```python
from build123d import *

# Parameters (mm, degrees)
CONG_1_R                     = 1
ENL_V_MAT_EXTRU_1_REACH      = 29.308
R_P_TITION_CIRCULAIRE2_COUNT = 3
R_P_TITION_CIRCULAIRE2_ANGLE = 180
ENL_V_START                  = -3.5
ENL_V_MAT_EXTRU_2_DEPTH      = 3.5
TROU_TARAUD_M3X0_52_D        = 2.5


with BuildPart() as part:
    # Esquisse3 → Révolution1 (revolve)
    with BuildSketch(Plane.XY):
        Polygon((-12.974994046, -8.820980619), (-12.974994046, -3.820980619), (-11.974994046, -3.820980619), (-11.974994046, -5.320980619), (-4.974994046, -5.320980619), (-4.974994046, -3.320980619), (-3.974994046, -3.320980619), (-3.974994046, 9.179019381), (-2.974994046, 9.179019381), (-2.974994046, 5.770549628), (-1.974994046, 5.770549628), (-1.974994046, -4.820980619), (-2.974994046, -4.820980619), (-2.974994046, -8.820980619), align=None)
    revolve(axis=Axis((1.025005954, 13.743921907, 0), (0, -1, 0)))

    # Congé1
    cong_1_edges = [part.edges().sort_by_distance(p)[0] for p in [
        (15.025005954, -8.820980619, 0),
    ]]
    fillet(cong_1_edges, radius=CONG_1_R)

    # Enlèv. mat.-Extru.1: up to this face of the body (flat: up to its plane)
    enl_v_mat_extru_1_end = Plane(part.part.faces().sort_by_distance((13.657310428, -5.320980619, 0))[0])
    # Esquisse5 → Enlèv. mat.-Extru.1 (cut, up to the picked face)
    with BuildSketch(Plane.XZ.offset(8.820980619), mode=Mode.PRIVATE) as enl_v_mat_extru_1_sk1:
        with BuildLine():
            Line((13.674116595, 3), (10.546683691, 3))
            ThreePointArc((10.546683691, 3), (7.546683691, 0), (10.546683691, -3))
            Line((10.546683691, -3), (13.674116595, -3))
            Line((13.674116595, -3), (14.699800285, -3))
            Line((14.699800285, -3), (15.031061769, -3))
            ThreePointArc((15.031061769, -3), (15.351470019, 0), (15.031061769, 3))
            Line((15.031061769, 3), (14.699800285, 3))
            Line((14.699800285, 3), (13.674116595, 3))
        make_face()
    enl_v_mat_extru_1_tool1 = split(extrude(enl_v_mat_extru_1_sk1.sketch, amount=-ENL_V_MAT_EXTRU_1_REACH, mode=Mode.PRIVATE), bisect_by=enl_v_mat_extru_1_end, keep=Keep.BOTH, mode=Mode.PRIVATE)
    enl_v_mat_extru_1 = enl_v_mat_extru_1_tool1.solids().sort_by(Axis((11.686689, -8.820981, 0), (0, 1, 0)))[0]
    add(enl_v_mat_extru_1, mode=Mode.SUBTRACT)

    # Répétition circulaire2: Enlèv. mat.-Extru.1 ×3 about axis
    r_p_tition_circulaire2_axis = Axis((1.025005954, 0, 0), (0, 1, 0))
    for i in range(1, R_P_TITION_CIRCULAIRE2_COUNT):
        add(enl_v_mat_extru_1.rotate(r_p_tition_circulaire2_axis, i * R_P_TITION_CIRCULAIRE2_ANGLE / (R_P_TITION_CIRCULAIRE2_COUNT - 1)), mode=Mode.SUBTRACT)

    # Esquisse7 → Enlèv. mat.-Extru.2 (cut)
    with BuildSketch(Plane.XZ.offset(8.820980619).offset(ENL_V_START)):
        with BuildLine():
            Line((-3.356038211, 12.2395446), (-1.541479015, 8.2395446))
            ThreePointArc((-1.541479015, 8.2395446), (0.968033239, 6.591412228), (3.533049808, 8.151759008))
            Line((3.533049808, 8.151759008), (5.643961789, 12.151759008))
            Line((5.643961789, 12.151759008), (6.71991785, 14.19060491))
            ThreePointArc((6.71991785, 14.19060491), (1.235603593, 15.289242553), (-4.276890033, 14.34207754))
            Line((-4.276890033, 14.34207754), (-3.356038211, 12.2395446))
        make_face()
    extrude(amount=ENL_V_MAT_EXTRU_2_DEPTH, mode=Mode.SUBTRACT)

    # Trou taraudé M3x0.52 (through all)
    with Locations(Plane(origin=(-5.37489391, -5.320980619, 6.540737726), x_dir=(1, 0, 0), z_dir=(0, 1, 0))):
        with Locations((0, 0), (1.060660172, 12.02081528), (12.020815281, 1.060660172), (13.081475452, 13.081475452)):
            Hole(TROU_TARAUD_M3X0_52_D / 2)


solid = part.part
```
Model file for the job. Use its own axes, mm. A direction names the side the tool comes from. Give positions to 0.01 mm unless a question says otherwise; leave off trailing zeros. Loops run counter-clockwise (first coordinate to the right, second up) from the corner with the lowest first, then second, coordinate; pieces in that order, holes last. Notation, with made-up numbers: (56.25, 79) - (74.25, 79) arc R24 ccw to (74.25, 113) - close; hole circle Ø1 at (13, 71.25). An arc over 180 degrees is marked (long way). One line per item, written item: value. Start each with the question number.
1. Slice it at A-A (z = 0). Give the number of separate pieces and of enclosed holes in the cut face, plus the area to 3 significant figures.
2. Pin check, flat tips, straight feed: pin 1 (2.5 mm diameter, centred on x = -0.5, z = 0.5, fed in from -Y); pin 2 (1 mm diameter, centred on y = 2, z = -2, fed in from -X); pin 3 (1.1 mm diameter, centred on y = -8, z = -11, fed in from +X); pin 4 (1.8 mm diameter, centred on x = 13, y = -6, fed in from +Z). Stop position of each tip, or through.
3. Slice it at B-B (y = 1). List the corners of the cut face in (x, z) (3 decimals).
4. Slice it at D-D (y = -6.5). List the corners of the cut face in (x, z) (3 decimals), plus the area to 3 significant figures.
5. Which spindle directions (+Z, -Z, +X, -X, +Y, -Y) get a long thin tool onto all of the face, cutting with end or side? Do faces 1 (the flat face through (1.1, -5.321, 13.3)), 2 (the flat face through (-12.3, -5.321, 0)), 3 (the flat face through (13, -7, -3)), 4 (the flat face through (-1.975, -7, -12)). Say none if no direction does.
6. Pull direction X, two halves, no side cores. Call faces 5 (the cylindrical face through (4.022, 0.401, -0.132)), 6 (the cylindrical face through (-5.21, -7.1, 5.3)), 7 (the cylindrical face through (-11.91, -5.79, 5.36)), 8 (the flat face through (5, -3.321, -4)): pulls with the +X half, pulls with the -X half, needs draft (parallel to the pull), parting line crosses it, or undercut.
7. Probe L1, parallel to X at y = -4.5, z = 1.75; L2, parallel to Y at x = 5.25, z = -11; L3, parallel to Y at x = -6.5, z = -11.5. List the from-to ranges inside material, lowest first. Write a range as from..to.
Solution:
1. separate pieces: 4
1. enclosed holes: 0
1. area: 74.8 mm^2
2. pin 1: passes through
2. pin 2: stops at x = -3.74
2. pin 3: stops at x = 10.33
2. pin 4: stops at z = 8.56
3. outline: circle Ø10 at (1.025, 0); hole circle Ø6 at (1.025, 0)
4. outline: (-12.65, -3) arc R14 ccw to (-1.975, -13.675) - (-1.975, -9.522) arc R3 cw to (4.025, -9.522) - (4.025, -13.675) arc R14 ccw to (14.7, -3) - (10.547, -3) arc R3 cw to (10.547, 3) - (14.7, 3) arc R14 ccw to (6.114, 13.042) - (3.533, 8.152) arc R2.809 cw to (-1.541, 8.24) - (-3.356, 12.24) - (-3.758, 13.158) arc R14 ccw to (-12.65, 3) - (-8.497, 3) arc R3 cw to (-8.497, -3) - close; hole circle Ø2.5 at (-5.375, 6.541); hole circle Ø2.5 at (-4.314, -5.48); hole circle Ø8 at (1.025, 0); hole circle Ø2.5 at (6.646, 5.48); hole circle Ø2.5 at (7.707, -6.541)
4. area: 376 mm^2
5. face 1: +Z, -Y
5. face 2: -X, -Y
5. face 3: +X, -Y
5. face 4: -Z, -Y
6. face 5: undercut
6. face 6: undercut
6. face 7: parting line crosses it
6. face 8: needs draft
7. L1: x = -12.87..-11.86, -4.71..-1.41, 3.46..6.76, 13.91..14.92
7. L2: y = -8.82..-5.32
7. L3: y = -8.49..-3.82
